from build123d import *

# Parameters (mm, degrees)
SKETCH_1_W                 = 57.95
SKETCH_1_H                 = 49.98
COVER_2MM_DEPTH            = 2
SKETCH_2_R                 = 1.1
COVER_8XD2P2_THROUGH_DEPTH = 71.491027089


with BuildPart() as part:
    # 草图1 → Cover_2mm (new body)
    with BuildSketch(Plane.XY):
        with Locations((24.675, 20.69)):
            Rectangle(SKETCH_1_W, SKETCH_1_H)
    extrude(amount=COVER_2MM_DEPTH)


with BuildPart() as part_1:
    # Stock_Z_Position: moved
    add(part.part.moved(Location((0, 0, 11.1))))

    # 草图2 → Cover_8xD2p2_Through (cut, through all)
    with BuildSketch(Plane.XY.offset(13.1)):
        with Locations((-2.3, -1)):
            Circle(SKETCH_2_R)
        with Locations((-2.3, 43)):
            Circle(SKETCH_2_R)
        with Locations((51.65, -1)):
            Circle(SKETCH_2_R)
        with Locations((51.65, 43)):
            Circle(SKETCH_2_R)
        with Locations((12, -2.3)):
            Circle(SKETCH_2_R)
        with Locations((37.35, -2.3)):
            Circle(SKETCH_2_R)
        with Locations((3, 43.68)):
            Circle(SKETCH_2_R)
        with Locations((44, 43.68)):
            Circle(SKETCH_2_R)
    extrude(amount=-COVER_8XD2P2_THROUGH_DEPTH, mode=Mode.SUBTRACT)


solid = part_1.part
Geometry: final body of the model. Coordinates: model frame, mm. Round coordinates to 2 decimals unless told otherwise and drop trailing zeros. Write each loop counter-clockwise with the first axis right and the second up, starting at its lowest first coordinate (ties: lowest second). Pieces come first, ordered by that corner, then holes. Notation, with made-up numbers: M 41,63 L 46,63 A32 cw 46,102 Z; hole C 82.5,68.5 d5. An arc over 180 degrees is marked long. Write item = value, one per line.
Item 1: Material intervals for line 1 along Y through (x, z) = (-2.3, 12.3); line 2 along Y through (x, z) = (44, 12.6); line 3 along Y through (x, z) = (12, 12.5), sorted ascending. Write a range as [from, to].
Findings:
line_1 = [-4.3, -2.1], [0.1, 41.9], [44.1, 45.68]
line_2 = [-4.3, 42.58], [44.78, 45.68]
line_3 = [-4.3, -3.4], [-1.2, 45.68]
Item 2: Pull-direction query (X, two-part tool) for faces 1 (the face through (-3.4, -1, 12.1)), 2 (the face through (-4.3, 20, 12)), 3 (the face through (24, 45.68, 12)); classes: pulls with the +X half, pulls with the -X half, needs draft (parallel to the pull), parting line crosses it, or undercut.
Findings:
face_1 = undercut
face_2 = pulls with the -X half
face_3 = needs draft
Item 3: Section query A-A on x = -2.3. Return loops of the section in (y, z).
Findings:
outline = M -4.3,11.1 L -2.1,11.1 L -2.1,13.1 L -4.3,13.1 Z; M 0.1,11.1 L 41.9,11.1 L 41.9,13.1 L 0.1,13.1 Z; M 44.1,11.1 L 45.68,11.1 L 45.68,13.1 L 44.1,13.1 Z
Item 4: Pin query (flat end, axial travel): P1, Ø1.8, axis at x = 3, y = 43.68, coming from the -Z side; P2, Ø3, axis at x = -2.3, y = 43, coming from the -Z side. Return the tip coordinate at first contact, or that it passes through.
Findings:
P1 = through
P2 = 11.1
